Geometry check sheet. Reference: the model listing, model coordinates, mm. Coordinates: 2 decimals unless noted, no trailing zeros. Loops run counter-clockwise (first coordinate to the right, second up) from the corner with the lowest first, then second, coordinate; pieces in that order, holes last.
from build123d import *

# Parameters (mm, degrees)
ESQUISSE1_W             = 24.82
ESQUISSE1_H             = 44
ESQUISSE1_R             = 1.5
BOSS_EXTRU_1_DEPTH      = 6
ESQUISSE2_R             = 1.175
ENL_V_MAT_EXTRU_1_DEPTH = 6


with BuildPart() as part:
    # Esquisse1 → Boss.-Extru.1 (new body)
    with BuildSketch(Plane.XY):
        with Locations((-51.605872064, 20.185897225)):
            Rectangle(ESQUISSE1_W, ESQUISSE1_H)
        with Locations((-60.605872064, 1.185897225)):
            Circle(ESQUISSE1_R, mode=Mode.SUBTRACT)
        with Locations((-42.605872064, 1.185897225)):
            Circle(ESQUISSE1_R, mode=Mode.SUBTRACT)
    extrude(amount=BOSS_EXTRU_1_DEPTH)

    # Esquisse2 → Enlèv. mat.-Extru.1 (cut)
    with BuildSketch(Plane.XY.offset(6)):
        with Locations((-43.605872064, 31.185897225)):
            Circle(ESQUISSE2_R)
        with Locations((-59.605872064, 31.185897225)):
            Circle(ESQUISSE2_R)
        with Locations((-59.605872064, 15.185897225)):
            Circle(ESQUISSE2_R)
        with Locations((-43.605872064, 15.185897225)):
            Circle(ESQUISSE2_R)
    extrude(amount=-ENL_V_MAT_EXTRU_1_DEPTH, mode=Mode.SUBTRACT)


solid = part.part
1) Depth check by flat-ended pin: pin 1 (2 mm diameter, centred on x = -52.5, y = 5.5, fed in from -Z); pin 2 (2.5 mm diameter, centred on x = -42.61, y = 1.19, fed in from +Z). Enter the tip coordinate at first touch or a pass-through.
Data:
pin 1: stops at z = 0
pin 2: passes through
2) Section check A-A on x = -59.75. Record the cut outline in (y, z), and give its area (3 significant figures).
Data:
outline: (-1.81, 0) - (-0.05, 0) - (-0.05, 6) - (-1.81, 6) - close; (2.42, 0) - (14.02, 0) - (14.02, 6) - (2.42, 6) - close; (16.35, 0) - (30.02, 0) - (30.02, 6) - (16.35, 6) - close; (32.35, 0) - (42.19, 0) - (42.19, 6) - (32.35, 6) - close
area: 221 mm2
3) Material ranges on probe 1 along Y at (x, z) = (-43, 1.3); probe 2 along X at (y, z) = (1, 2.5); probe 3 along X at (y, z) = (31, 5.15), recorded low to high.
Data:
probe 1: y = -1.81 to -0.26, 2.63 to 14.18, 16.19 to 30.18, 32.19 to 42.19
probe 2: x = -64.02 to -62.09, -59.12 to -44.09, -41.12 to -39.2
probe 3: x = -64.02 to -60.77, -58.45 to -44.77, -42.45 to -39.2
4) Section check B-B on z = 2.75. Record the cut outline in (x, y) (3 decimals).
Data:
outline: (-64.016, -1.814) - (-39.196, -1.814) - (-39.196, 42.186) - (-64.016, 42.186) - close; hole circle Ø3 at (-60.606, 1.186); hole circle Ø2.35 at (-59.606, 15.186); hole circle Ø2.35 at (-59.606, 31.186); hole circle Ø2.35 at (-43.606, 15.186); hole circle Ø2.35 at (-43.606, 31.186); hole circle Ø3 at (-42.606, 1.186)
5) Mould release check, pull along Y, two halves, no side actions. Record for faces 1 (the cylindrical face through (-58.52, 30.74, 3.04)), 2 (the flat face through (-52, 42.186, 3)), 3 (the flat face through (-52, 20, 0)), 4 (the cylindrical face through (-58.485, 15.539, 3.042)): +Y half, -Y half, draft (parallel to the pull), parting line (faces both ways), or undercut.
Data:
face 1: undercut
face 2: +Y half
face 3: draft
face 4: undercut
